Study the drawing (mm; zero at the part's minimum x, y, z) and answer. A direction names the side the tool comes from. Round coordinates to 2 decimals unless told otherwise and drop trailing zeros. Loops run counter-clockwise (first coordinate to the right, second up) from the corner with the lowest first, then second, coordinate; pieces in that order, holes last. Notation, with made-up numbers: (-27.5, 18) -> (-9.5, 18) arc R14 cw to (-9.5, 30) -> close; hole circle Ø2 at (-17, 12). An arc over 180 degrees is marked (long way). Use one line per item in the form item = value.
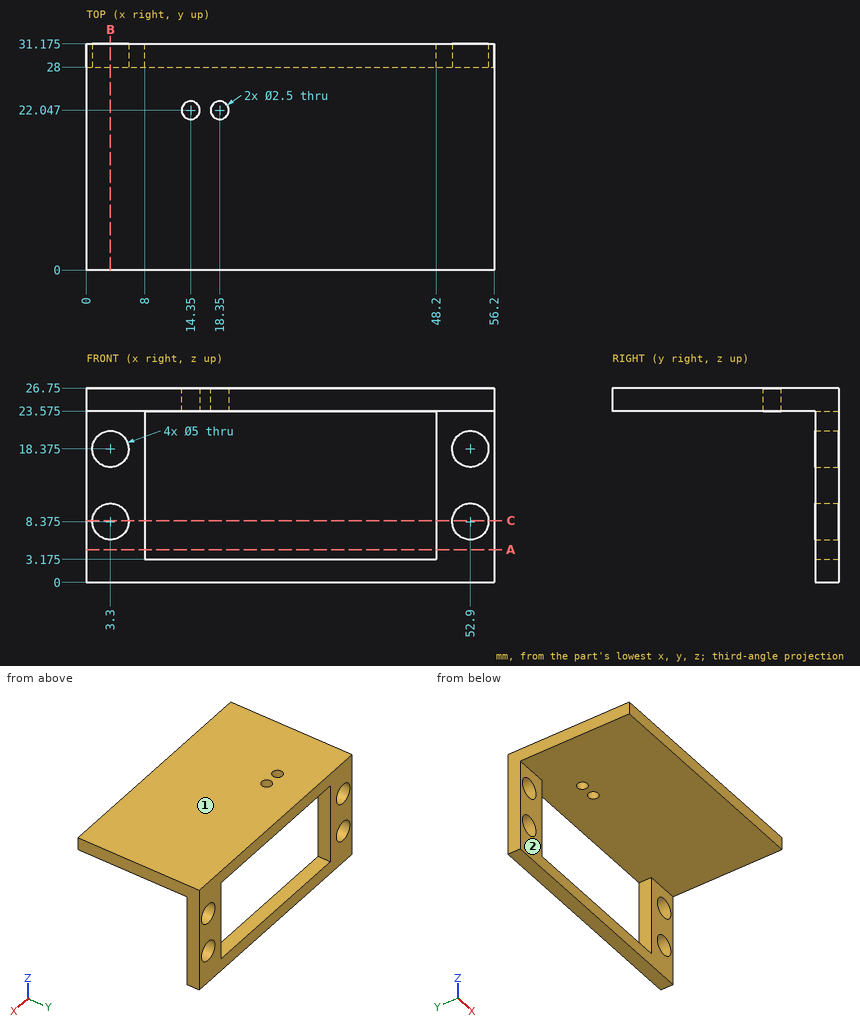
(1) For the marked faces 1 and 2, determine the directions among +Z, -Z, +X, -X, +Y, -Y from which every point of the face is accessible in a straight line to the end or side of a thin tool.
Completed:
face_1 = +Z, +X, -X, +Y, -Y
face_2 = -Z, +X, -X, -Y
(2) Find section B-B, the plane x = 3.3. State how many separate pieces and enclosed holes the cut face has, then the cut area to 3 significant figures.
Completed:
separate_pieces = 3
enclosed_holes = 0
area = 142 mm2
(3) Find section C-C, the plane z = 8.5. Write down the section's boundary in (x, y) (1 decimal).
Completed:
outline = (0, 28) -> (0.8, 28) -> (0.8, 31.2) -> (0, 31.2) -> close; (5.8, 28) -> (8, 28) -> (8, 31.2) -> (5.8, 31.2) -> close; (48.2, 28) -> (50.4, 28) -> (50.4, 31.2) -> (48.2, 31.2) -> close; (55.4, 28) -> (56.2, 28) -> (56.2, 31.2) -> (55.4, 31.2) -> close
(4) Given P1, Ø3.5, axis at y = 29, z = 12, coming from the -X side; P2, Ø8, axis at x = 3.3, z = 8.375, coming from the -Y side; P3, Ø4, axis at x = 14.35, y = 22.05, coming from the -Z side (3 decimals), each flat-ended and moving along its own axis, determine where each tip first touches the part or whether it passes through.
Completed:
P1 = 0
P2 = 28
P3 = 23.575
(5) Find section A-A, the plane z = 4.5. Write down the section's boundary in (x, y) (1 decimal).
Completed:
outline = (0, 28) -> (8, 28) -> (8, 31.2) -> (0, 31.2) -> close; (48.2, 28) -> (56.2, 28) -> (56.2, 31.2) -> (48.2, 31.2) -> close
(6) Consider L1, parallel to Y at x = 14.35, z = 25.6 (1 decimal); L2, parallel to Y at x = 18, z = 24.5 (1 decimal). Determine where each line is inside the solid, lowest interval first.
Completed:
L1 = 0 to 20.8, 23.3 to 31.2
L2 = 0 to 20.8, 23.2 to 31.2
